Autodesk Inventor part; units mm, degrees
ref_plane "a1_XY" through (0, 8.7376, -14.1351) normal (0, 1, 0) x (1, 0, 0)
ref_plane "a1_YZ" through (0, 8.7376, -14.1351) normal (1, 0, 0) x (0, 0, -1)
ref_plane "a1_ZX" through (0, 8.7376, -14.1351) normal (0, 0, -1) x (0, 1, 0)
sketch "Sketch_1" plane through (0, 0, 0) normal (0, 0, 1) x (1, 0, 0)
  line L0 (0, 0) -> (0, 8.7376)
  line L1 (0, 8.7376) -> (14.1351, 8.7376)
  line L2 (14.1351, 8.7376) -> (14.1351, 0)
  line L3 (14.1351, 0) -> (0, 0)
  line L4 (0, 0) -> (0, 8.7376)
revolve "Revolution1" add sketch "Sketch_1" angle 360 about axis through (0, 0, 0) along (0, -1, 0)
sketch "Sketch_63" plane through (0, 0, 0) normal (0, 1, 0) x (-1, 0, 0)
  line L0 (20.6184, 14.1351) -> (13.5509, 14.1351)
  line L1 (13.5509, 14.1351) -> (13.5509, -14.1351)
  line L2 (13.5509, -14.1351) -> (20.6184, -14.1351)
  line L3 (20.6184, -14.1351) -> (20.6184, 14.1351)
extrude "Extrusion1" cut sketch "Sketch_63" along normal blind 8.7376
sketch "Sketch_37" plane through (0, 0, 0) normal (0, 0, 1) x (1, 0, 0)
  line L0 (-5.8778, 4.3688) -> (-14.1351, 4.3688)
  line L1 (-14.1351, 4.3688) -> (-14.1351, 8.3376)
  line L2 (-14.1351, 8.3376) -> (-13.5509, 8.3376)
  line L3 (-13.5509, 8.3376) -> (-13.5509, 6.7818)
  line L4 (-13.5509, 6.7818) -> (-13.1216, 6.3525)
  line L5 (-13.1216, 6.3525) -> (-7.0231, 6.3525)
  line L6 (-7.0231, 6.3525) -> (-5.8778, 4.3688)
  line L7 (-5.8778, 4.3688) -> (-14.1351, 4.3688)
revolve "Revolution2" cut sketch "Sketch_37" angle 360 about axis through (-5.8778, 4.3688, 0) along (1, 0, 0)
thread "Thread1"
sketch "Sketch4" plane through (0, 0, 0) normal (0, -1, 0) x (1, 0, 0)
  point P0 (0, 0)
hole "Hole1" at (0, 0, 0) direction (0, 1, 0) diameter 6.4008 depth 8.7376
sketch "Sketch_9" plane through (0, 0, 0) normal (0, 0, 1) x (1, 0, 0)
  line L0 (0, 0) -> (0, 2.54)
  line L1 (0, 2.54) -> (7.747, 2.54)
  line L2 (7.747, 2.54) -> (7.747, 0)
  line L3 (7.747, 0) -> (0, 0)
  line L4 (0, 0) -> (0, 2.54)
revolve "Revolution3" cut sketch "Sketch_9" angle 360 about axis through (0, 0, 0) along (0, -1, 0)
sketch "Sketch6" plane through (0, 8.7376, 0) normal (0, 1, 0) x (1, 0, 0)
  point P0 (0, -11.1125)
hole "Hole2" at (0, 8.7376, 11.1125) direction (0, -1, 0) diameter 3.2639 depth 8.7376 counterbore diameter 5.08 counterbore depth 3.048
sketch "Sketch7" plane through (0, 8.7376, 0) normal (0, 1, 0) x (1, 0, 0)
  point P0 (0, 11.1125)
hole "Hole3" at (0, 8.7376, -11.1125) direction (0, -1, 0) diameter 3.2639 depth 8.7376 counterbore diameter 5.08 counterbore depth 3.048
sketch "Sketch8" plane through (0, 8.7376, 0) normal (0, 1, 0) x (1, 0, 0)
  point P0 (-7.7589, 7.7589)
hole "Hole4" at (-7.7589, 8.7376, -7.7589) direction (0, -1, 0) diameter 3.2639 depth 8.7376 counterbore diameter 5.08 counterbore depth 3.81
pattern_linear "Rectangular Pattern1" count 2 spacing 15.5179 along (1, 0, 0) count 2 spacing 15.5179 along (0, 0, 1) of "Hole4"
ref_plane "a1_XY" through (0, 8.7376, -14.1351) normal (0, 1, 0) x (1, 0, 0)
ref_plane "a1_YZ" through (0, 8.7376, -14.1351) normal (1, 0, 0) x (0, 0, -1)
ref_plane "a1_ZX" through (0, 8.7376, -14.1351) normal (0, 0, -1) x (0, 1, 0)
ref_plane "a2_XY" through (0, 8.7376, 14.1351) normal (0, 1, 0) x (1, 0, 0)
ref_plane "a2_YZ" through (0, 8.7376, 14.1351) normal (1, 0, 0) x (0, 0, -1)
ref_plane "a2_ZX" through (0, 8.7376, 14.1351) normal (0, 0, -1) x (0, 1, 0)
ref_plane "ab_tr1_XY" through (-7.5198, 0, -2.0149) normal (0, 1, 0) x (1, 0, 0)
ref_plane "ab_tr1_YZ" through (-7.5198, 0, -2.0149) normal (1, 0, 0) x (0, 0, -1)
ref_plane "ab_tr1_ZX" through (-7.5198, 0, -2.0149) normal (0, 0, -1) x (0, 1, 0)
ref_plane "ab_tr2_XY" through (7.5198, 0, 2.0149) normal (0, 1, 0) x (1, 0, 0)
ref_plane "ab_tr2_YZ" through (7.5198, 0, 2.0149) normal (1, 0, 0) x (0, 0, -1)
ref_plane "ab_tr2_ZX" through (7.5198, 0, 2.0149) normal (0, 0, -1) x (0, 1, 0)
ref_plane "ab_tr3_XY" through (-2.0149, 0, 7.5198) normal (0, 1, 0) x (1, 0, 0)
ref_plane "ab_tr3_YZ" through (-2.0149, 0, 7.5198) normal (1, 0, 0) x (0, 0, -1)
ref_plane "ab_tr3_ZX" through (-2.0149, 0, 7.5198) normal (0, 0, -1) x (0, 1, 0)
ref_plane "ab_tr4_XY" through (2.0149, 0, -7.5198) normal (0, 1, 0) x (1, 0, 0)
ref_plane "ab_tr4_YZ" through (2.0149, 0, -7.5198) normal (1, 0, 0) x (0, 0, -1)
ref_plane "ab_tr4_ZX" through (2.0149, 0, -7.5198) normal (0, 0, -1) x (0, 1, 0)
ref_plane "ar3_XY" through (-7.9026, 2.54, 7.9026) normal (0, 1, 0) x (1, 0, 0)
ref_plane "ar3_YZ" through (-7.9026, 2.54, 7.9026) normal (1, 0, 0) x (0, 0, -1)
ref_plane "ar3_ZX" through (-7.9026, 2.54, 7.9026) normal (0, 0, -1) x (0, 1, 0)
ref_plane "ar4_XY" through (7.9026, 2.54, 7.9026) normal (0, 1, 0) x (1, 0, 0)
ref_plane "ar4_YZ" through (7.9026, 2.54, 7.9026) normal (1, 0, 0) x (0, 0, -1)
ref_plane "ar4_ZX" through (7.9026, 2.54, 7.9026) normal (0, 0, -1) x (0, 1, 0)
ref_plane "ar5_XY" through (7.9026, 2.54, -7.9026) normal (0, 1, 0) x (1, 0, 0)
ref_plane "ar5_YZ" through (7.9026, 2.54, -7.9026) normal (1, 0, 0) x (0, 0, -1)
ref_plane "ar5_ZX" through (7.9026, 2.54, -7.9026) normal (0, 0, -1) x (0, 1, 0)
ref_plane "ar6_XY" through (-7.9026, 2.54, -7.9026) normal (0, 1, 0) x (1, 0, 0)
ref_plane "ar6_YZ" through (-7.9026, 2.54, -7.9026) normal (1, 0, 0) x (0, 0, -1)
ref_plane "ar6_ZX" through (-7.9026, 2.54, -7.9026) normal (0, 0, -1) x (0, 1, 0)
ref_plane "b1_XY" through (0, 8.7376, 0) normal (0, 1, 0) x (1, 0, 0)
ref_plane "b1_YZ" through (0, 8.7376, 0) normal (1, 0, 0) x (0, 0, -1)
ref_plane "b1_ZX" through (0, 8.7376, 0) normal (0, 0, -1) x (0, 1, 0)
ref_plane "j_XY" through (0, 0, 0) normal (0, 1, 0) x (1, 0, 0)
ref_plane "j_YZ" through (0, 0, 0) normal (1, 0, 0) x (0, 0, -1)
ref_plane "j_ZX" through (0, 0, 0) normal (0, 0, -1) x (0, 1, 0)
ref_plane "k1_XY" through (-13.5509, 4.3688, 0) normal (0, 0, 1) x (1, 0, 0)
ref_plane "k1_YZ" through (-13.5509, 4.3688, 0) normal (1, 0, 0) x (0, 1, 0)
ref_plane "k1_ZX" through (-13.5509, 4.3688, 0) normal (0, 1, 0) x (0, 0, 1)
ref_plane "k2_XY" through (-13.5509, 8.7376, 0) normal (0, 0, 1) x (1, 0, 0)
ref_plane "k2_YZ" through (-13.5509, 8.7376, 0) normal (1, 0, 0) x (0, 1, 0)
ref_plane "k2_ZX" through (-13.5509, 8.7376, 0) normal (0, 1, 0) x (0, 0, 1)
ref_plane "l1_XY" through (-13.5509, 6.7818, 0) normal (0, 0, 1) x (1, 0, 0)
ref_plane "l1_YZ" through (-13.5509, 6.7818, 0) normal (1, 0, 0) x (0, 1, 0)
ref_plane "l1_ZX" through (-13.5509, 6.7818, 0) normal (0, 1, 0) x (0, 0, 1)
ref_plane "l2_XY" through (-13.5509, 1.9558, 0) normal (0, 0, 1) x (1, 0, 0)
ref_plane "l2_YZ" through (-13.5509, 1.9558, 0) normal (1, 0, 0) x (0, 1, 0)
ref_plane "l2_ZX" through (-13.5509, 1.9558, 0) normal (0, 1, 0) x (0, 0, 1)
ref_plane "nut_XY" through (0, 15.9766, 0) normal (0, 1, 0) x (1, 0, 0)
ref_plane "nut_YZ" through (0, 15.9766, 0) normal (1, 0, 0) x (0, 0, -1)
ref_plane "nut_ZX" through (0, 15.9766, 0) normal (0, 0, -1) x (0, 1, 0)
ref_plane "po1_XY" through (7.7589, 0, 7.7589) normal (0, 1, 0) x (1, 0, 0)
ref_plane "po1_YZ" through (7.7589, 0, 7.7589) normal (1, 0, 0) x (0, 0, -1)
ref_plane "po1_ZX" through (7.7589, 0, 7.7589) normal (0, 0, -1) x (0, 1, 0)
ref_plane "po2_XY" through (7.7589, 0, -7.7589) normal (0, 1, 0) x (1, 0, 0)
ref_plane "po2_YZ" through (7.7589, 0, -7.7589) normal (1, 0, 0) x (0, 0, -1)
ref_plane "po2_ZX" through (7.7589, 0, -7.7589) normal (0, 0, -1) x (0, 1, 0)
ref_plane "po3_XY" through (-7.7589, 0, -7.7589) normal (0, 1, 0) x (1, 0, 0)
ref_plane "po3_YZ" through (-7.7589, 0, -7.7589) normal (1, 0, 0) x (0, 0, -1)
ref_plane "po3_ZX" through (-7.7589, 0, -7.7589) normal (0, 0, -1) x (0, 1, 0)
ref_plane "po4_XY" through (-7.7589, 0, 7.7589) normal (0, 1, 0) x (1, 0, 0)
ref_plane "po4_YZ" through (-7.7589, 0, 7.7589) normal (1, 0, 0) x (0, 0, -1)
ref_plane "po4_ZX" through (-7.7589, 0, 7.7589) normal (0, 0, -1) x (0, 1, 0)
ref_plane "r7_XY" through (1.7526, 8.7376, 11.1125) normal (0, 1, 0) x (1, 0, 0)
ref_plane "r7_YZ" through (1.7526, 8.7376, 11.1125) normal (1, 0, 0) x (0, 0, -1)
ref_plane "r7_ZX" through (1.7526, 8.7376, 11.1125) normal (0, 0, -1) x (0, 1, 0)
ref_plane "r71_XY" through (0, 8.7376, 11.1125) normal (0, 1, 0) x (1, 0, 0)
ref_plane "r71_YZ" through (0, 8.7376, 11.1125) normal (1, 0, 0) x (0, 0, -1)
ref_plane "r71_ZX" through (0, 8.7376, 11.1125) normal (0, 0, -1) x (0, 1, 0)
ref_plane "r72_XY" through (-1.7526, 8.7376, 11.1125) normal (0, 1, 0) x (1, 0, 0)
ref_plane "r72_YZ" through (-1.7526, 8.7376, 11.1125) normal (1, 0, 0) x (0, 0, -1)
ref_plane "r72_ZX" through (-1.7526, 8.7376, 11.1125) normal (0, 0, -1) x (0, 1, 0)
ref_plane "r73_XY" through (0, 8.7376, -11.1125) normal (0, 1, 0) x (1, 0, 0)
ref_plane "r73_YZ" through (0, 8.7376, -11.1125) normal (1, 0, 0) x (0, 0, -1)
ref_plane "r73_ZX" through (0, 8.7376, -11.1125) normal (0, 0, -1) x (0, 1, 0)
ref_plane "rg_XY" through (0, 8.7376, 0) normal (0, 1, 0) x (1, 0, 0)
ref_plane "rg_YZ" through (0, 8.7376, 0) normal (1, 0, 0) x (0, 0, -1)
ref_plane "rg_ZX" through (0, 8.7376, 0) normal (0, 0, -1) x (0, 1, 0)
ref_plane "rh_XY" through (0, 8.7376, 0) normal (0, 1, 0) x (1, 0, 0)
ref_plane "rh_YZ" through (0, 8.7376, 0) normal (1, 0, 0) x (0, 0, -1)
ref_plane "rh_ZX" through (0, 8.7376, 0) normal (0, 0, -1) x (0, 1, 0)
ref_plane "rs_1_XY" through (0, 10.5156, -11.1125) normal (0, 1, 0) x (1, 0, 0)
ref_plane "rs_1_YZ" through (0, 10.5156, -11.1125) normal (1, 0, 0) x (0, 0, -1)
ref_plane "rs_1_ZX" through (0, 10.5156, -11.1125) normal (0, 0, -1) x (0, 1, 0)
ref_plane "rs_2_XY" through (-11.1125, 10.5156, 0) normal (0, 1, 0) x (1, 0, 0)
ref_plane "rs_2_YZ" through (-11.1125, 10.5156, 0) normal (1, 0, 0) x (0, 0, -1)
ref_plane "rs_2_ZX" through (-11.1125, 10.5156, 0) normal (0, 0, -1) x (0, 1, 0)
ref_plane "rs_3_XY" through (0, 10.5156, 11.1125) normal (0, 1, 0) x (1, 0, 0)
ref_plane "rs_3_YZ" through (0, 10.5156, 11.1125) normal (1, 0, 0) x (0, 0, -1)
ref_plane "rs_3_ZX" through (0, 10.5156, 11.1125) normal (0, 0, -1) x (0, 1, 0)
ref_plane "rs_4_XY" through (11.1125, 10.5156, 0) normal (0, 1, 0) x (1, 0, 0)
ref_plane "rs_4_YZ" through (11.1125, 10.5156, 0) normal (1, 0, 0) x (0, 0, -1)
ref_plane "rs_4_ZX" through (11.1125, 10.5156, 0) normal (0, 0, -1) x (0, 1, 0)
ref_plane "sc1_XY" through (7.7589, 4.9276, -7.7589) normal (0, 1, 0) x (1, 0, 0)
ref_plane "sc1_YZ" through (7.7589, 4.9276, -7.7589) normal (1, 0, 0) x (0, 0, -1)
ref_plane "sc1_ZX" through (7.7589, 4.9276, -7.7589) normal (0, 0, -1) x (0, 1, 0)
ref_plane "sc2_XY" through (-7.7589, 4.9276, -7.7589) normal (0, 1, 0) x (1, 0, 0)
ref_plane "sc2_YZ" through (-7.7589, 4.9276, -7.7589) normal (1, 0, 0) x (0, 0, -1)
ref_plane "sc2_ZX" through (-7.7589, 4.9276, -7.7589) normal (0, 0, -1) x (0, 1, 0)
ref_plane "sc3_XY" through (-7.7589, 4.9276, 7.7589) normal (0, 1, 0) x (1, 0, 0)
ref_plane "sc3_YZ" through (-7.7589, 4.9276, 7.7589) normal (1, 0, 0) x (0, 0, -1)
ref_plane "sc3_ZX" through (-7.7589, 4.9276, 7.7589) normal (0, 0, -1) x (0, 1, 0)
ref_plane "sc4_XY" through (7.7589, 4.9276, 7.7589) normal (0, 1, 0) x (1, 0, 0)
ref_plane "sc4_YZ" through (7.7589, 4.9276, 7.7589) normal (1, 0, 0) x (0, 0, -1)
ref_plane "sc4_ZX" through (7.7589, 4.9276, 7.7589) normal (0, 0, -1) x (0, 1, 0)
ref_plane "to_dummy_XY" through (0, 8.7376, 0) normal (0, 1, 0) x (1, 0, 0)
ref_plane "to_dummy_YZ" through (0, 8.7376, 0) normal (1, 0, 0) x (0, 0, -1)
ref_plane "to_dummy_ZX" through (0, 8.7376, 0) normal (0, 0, -1) x (0, 1, 0)
ref_plane "to_nut_XY" through (0, 10.3124, 0) normal (0, 1, 0) x (1, 0, 0)
ref_plane "to_nut_YZ" through (0, 10.3124, 0) normal (1, 0, 0) x (0, 0, -1)
ref_plane "to_nut_ZX" through (0, 10.3124, 0) normal (0, 0, -1) x (0, 1, 0)
ref_plane "to_rod_XY" through (0, 0, 0) normal (0, 1, 0) x (1, 0, 0)
ref_plane "to_rod_YZ" through (0, 0, 0) normal (1, 0, 0) x (0, 0, -1)
ref_plane "to_rod_ZX" through (0, 0, 0) normal (0, 0, -1) x (0, 1, 0)
ref_plane "to_tube_XY" through (0, 2.54, 0) normal (0, 1, 0) x (1, 0, 0)
ref_plane "to_tube_YZ" through (0, 2.54, 0) normal (1, 0, 0) x (0, 0, -1)
ref_plane "to_tube_ZX" through (0, 2.54, 0) normal (0, 0, -1) x (0, 1, 0)
ref_plane "to_wiper_XY" through (0, 8.7376, 0) normal (0, 1, 0) x (1, 0, 0)
ref_plane "to_wiper_YZ" through (0, 8.7376, 0) normal (1, 0, 0) x (0, 0, -1)
ref_plane "to_wiper_ZX" through (0, 8.7376, 0) normal (0, 0, -1) x (0, 1, 0)
ref_plane "track1_XY" through (-7.7851, 0, 0) normal (0, 1, 0) x (1, 0, 0)
ref_plane "track1_YZ" through (-7.7851, 0, 0) normal (1, 0, 0) x (0, 0, -1)
ref_plane "track1_ZX" through (-7.7851, 0, 0) normal (0, 0, -1) x (0, 1, 0)
ref_plane "track2_XY" through (0, 0, -7.7851) normal (0, 1, 0) x (1, 0, 0)
ref_plane "track2_YZ" through (0, 0, -7.7851) normal (1, 0, 0) x (0, 0, -1)
ref_plane "track2_ZX" through (0, 0, -7.7851) normal (0, 0, -1) x (0, 1, 0)
ref_plane "track3_XY" through (7.7851, 0, 0) normal (0, 1, 0) x (1, 0, 0)
ref_plane "track3_YZ" through (7.7851, 0, 0) normal (1, 0, 0) x (0, 0, -1)
ref_plane "track3_ZX" through (7.7851, 0, 0) normal (0, 0, -1) x (0, 1, 0)
ref_plane "track4_XY" through (0, 0, 7.7851) normal (0, 1, 0) x (1, 0, 0)
ref_plane "track4_YZ" through (0, 0, 7.7851) normal (1, 0, 0) x (0, 0, -1)
ref_plane "track4_ZX" through (0, 0, 7.7851) normal (0, 0, -1) x (0, 1, 0)
properties part number "02-1NT-0.125-FO1_BM_heads-bif"
Design review of the part built by this model. Coordinates are the model's own, in mm. A direction names the side the tool comes from. Give positions to 0.01 mm unless a question says otherwise; leave off trailing zeros. Loops run counter-clockwise (first coordinate to the right, second up) from the corner with the lowest first, then second, coordinate; pieces in that order, holes last. Notation, with made-up numbers: M 26.25,72 L 85.25,72 A26 cw 85.25,89 Z; hole C 75,39.5 d1. An arc over 180 degrees is marked long. Return JSON: item names as keys, results as strings. Group by question number.
Item 1: Insertion check: pin 1 Ø4 at (y, z) = (5.5, -6.5) entering from -X; pin 2 Ø2.5 at (x, z) = (1, 11.5) entering from +Y; pin 3 Ø5 at (y, z) = (4.5, 3.5) entering from +X. Each pin has a flat end and moves straight along its axis. Give the tip position at first contact, or say it passes through.
Item 2: We need section D-D (z = -5.75). Give the boundary of the cut face in (x, y).
Item 3: We need section B-B (x = 6.5). Give the boundary of the cut face in (y, z), and give its area (3 significant figures).
Item 4: Mouldability with a two-part tool opening along Y and no side actions: class faces 4 (the flat face through (2, 5.69, 11)), 5 (the cylindrical face through (-10.03, 6.26, 0.6)), 6 (the cylindrical face through (1.95, 5.68, 2.54)), 7 (the flat face through (3.35, 2.54, 0.11)) as released by +Y, released by -Y, zero draft, split by the parting line, or undercut.
Item 5: We need section C-C (x = 9.75). Give the boundary of the cut face in (y, z), and give its area (3 significant figures).
Item 6: Tool access review of faces 1 (the flat face through (-6, 4.928, 7)), 2 (the cylindrical face through (9.352, 2.429, -8.113)), 3 (the cylindrical face through (4.165, 1.252, 6.532)): name each direction out of +Z, -Z, +X, -X, +Y, -Y from which nothing blocks a thin tool from reaching the whole face with its end or side.
Item 7: We need section A-A (x = 0). Give the boundary of the cut face in (y, z).
Item 8: For probe 1 along Z at (x, y) = (0, 6.5); probe 2 along X at (y, z) = (1.2, 0); probe 3 along X at (y, z) = (4.25, 8.75), list the stretches that pass through material, from the lowest coordinate up.
Output:
{
 "1": {"pin 1": "stops at x = -13.4", "pin 2": "stops at y = 5.69", "pin 3": "stops at x = 14.1"},
 "2": {"outline": "M -12.91,0 L -5.19,0 L -5.19,2.54 L 5.19,2.54 L 5.19,0 L 12.91,0 L 12.91,8.74 L 9.31,8.74 L 9.31,4.93 L 6.2,4.93 L 6.2,8.74 L -6.2,8.74 L -6.2,4.93 L -9.31,4.93 L -9.31,8.74 L -12.91,8.74 Z"},
 "3": {"outline": "M 0,-12.55 L 8.74,-12.55 L 8.74,-9.96 L 4.93,-9.96 L 4.93,-8.8 L 0,-8.8 Z; M 0,-6.72 L 4.93,-6.72 L 4.93,-5.55 L 8.74,-5.55 L 8.74,5.55 L 4.93,5.55 L 4.93,6.72 L 0,6.72 L 0,4.21 L 2.54,4.21 L 2.54,-4.21 L 0,-4.21 Z; M 0,8.8 L 4.93,8.8 L 4.93,9.97 L 8.74,9.97 L 8.74,12.55 L 0,12.55 Z", "area": "144 mm^2"},
 "4": {"face 4": "released by +Y", "face 5": "undercut", "face 6": "zero draft", "face 7": "released by -Y"},
 "5": {"outline": "M 0,-10.23 L 8.74,-10.23 L 8.74,-9.34 L 4.93,-9.34 L 4.93,-6.18 L 8.74,-6.18 L 8.74,6.18 L 4.93,6.18 L 4.93,9.34 L 8.74,9.34 L 8.74,10.23 L 0,10.23 Z", "area": "155 mm^2"},
 "6": {"face 1": "+Y", "face 2": "+Y, -Y", "face 3": "-Y"},
 "7": {"outline": "M 0,-14.14 L 8.74,-14.14 L 8.74,-13.65 L 5.69,-13.65 L 5.69,-12.74 L 0,-12.74 Z; M 0,-9.48 L 5.69,-9.48 L 5.69,-8.57 L 8.74,-8.57 L 8.74,-3.2 L 2.54,-3.2 L 2.54,-7.75 L 0,-7.75 Z; M 0,7.75 L 2.54,7.75 L 2.54,3.2 L 8.74,3.2 L 8.74,8.57 L 5.69,8.57 L 5.69,9.48 L 0,9.48 Z; M 0,12.74 L 5.69,12.74 L 5.69,13.65 L 8.74,13.65 L 8.74,14.14 L 0,14.14 Z"},
 "8": {"probe 1": "z = -14.14 to -13.65, -8.57 to -3.2, 3.2 to 8.57, 13.65 to 14.14", "probe 2": "x = -13.55 to -7.75, 7.75 to 14.14", "probe 3": "x = -11.1 to -9.06, -6.46 to 6.46, 9.06 to 11.1"}
}
